Geometry check sheet. Reference: drawing and pictorial views, mm from the part's lowest x, y, z. A direction names the side the tool comes from. Coordinates: 2 decimals unless noted, no trailing zeros. Order: outer loops, then holes, each group sorted by start corner. A loop starts at its lowest first (then second) coordinate and runs counter-clockwise, first axis right, second up. Notation, with made-up numbers: (74.5, 64) -> (110.5, 64) arc R17 ccw to (110.5, 95) -> close; hole circle Ø7 at (-31.5, 80.25). An arc over 180 degrees is marked (long way). Use CSV: the item, a comma, the result in double quotes. Start each with the question number.
1) Tool access check on the marked faces 1, 2 and 3. Record the directions out of +Z, -Z, +X, -X, +Y, -Y that give a thin tool (end or side, any length) a straight path to the whole face; none if there is none.
2) Sectioned sample at A-A on z = 55.5. Give the number of separate pieces and of enclosed holes in the cut face, then the cut area to 3 significant figures.
3) Sectioned sample at C-C on x = 30. Record the boundary of the cut face in (y, z), then the cut area to 3 significant figures.
4) Scan lines: line 1 along X through (y, z) = (0.8, 19.5); line 2 along Z through (x, y) = (57.5, 2.1); line 3 along X through (y, z) = (1.25, 35.5). Record each from-to range of solid material in increasing order.
5) Sectioned sample at B-B on x = 57.5. Record the boundary of the cut face in (y, z).
6) Go/stop test with flat-tipped pins: pin 1 (4.5 mm diameter, centred on x = 55.5, z = 54, fed in from +Y); pin 2 (0.5 mm diameter, centred on y = 3.5, z = 47.5, fed in from +X); pin 3 (0.8 mm diameter, centred on y = 5, z = 26, fed in from +X). Record where each tip stops, or that it passes through.
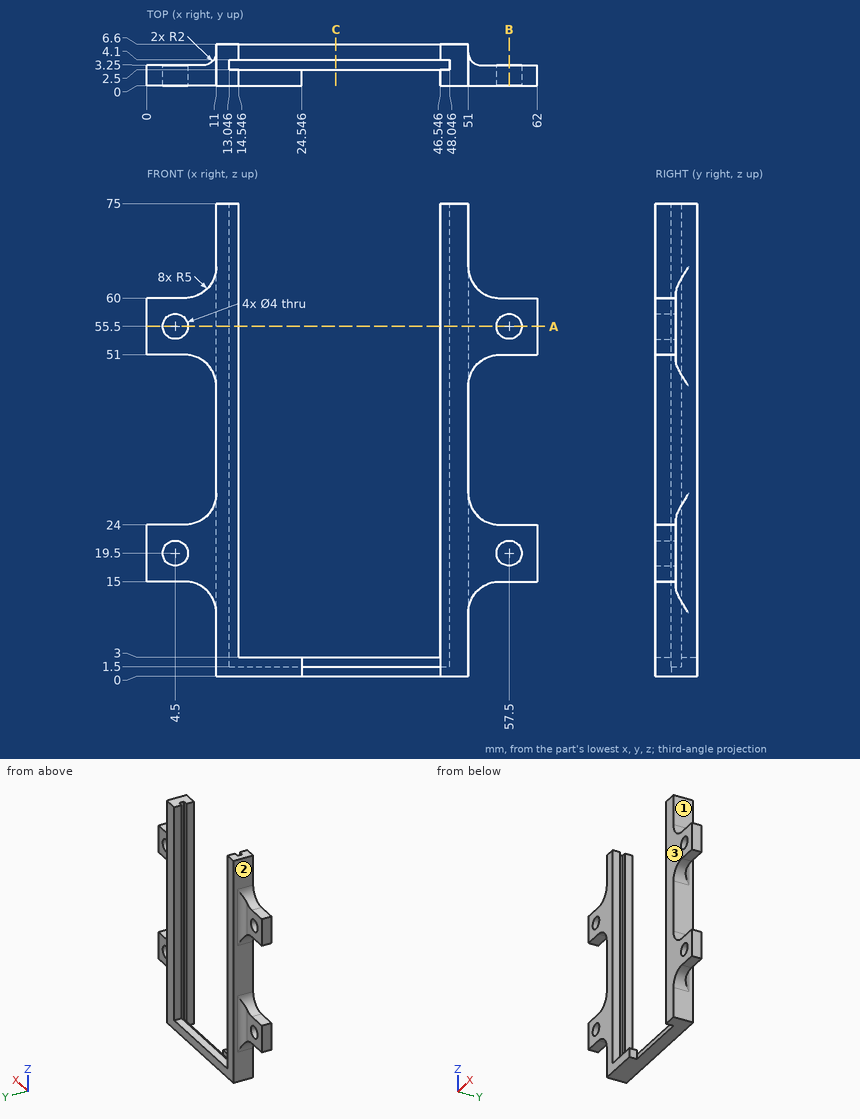
Answers follow:
1,face 1,"+X, +Y"
1,face 2,"-X, +Y"
1,face 3,"+Z, -Z, +X, -X, -Y"
2,separate pieces,"4"
2,enclosed holes,"0"
2,area,"95.2 mm²"
3,outline,"(2.5, 0) -> (6.6, 0) -> (6.6, 3) -> (4.1, 3) -> (4.1, 1.5) -> (2.5, 1.5) -> close"
3,area,"9.90 mm²"
4,line 1,"x = 0 to 2.5, 6.5 to 14.55, 46.55 to 55.5, 59.5 to 62"
4,line 2,"z = 15 to 17.5, 21.5 to 24, 51 to 53.5, 57.5 to 60"
4,line 3,"x = 11 to 14.55, 46.55 to 51"
5,outline,"(0, 15) -> (3.25, 15) -> (3.25, 17.5) -> (0, 17.5) -> close; (0, 21.5) -> (3.25, 21.5) -> (3.25, 24) -> (0, 24) -> close; (0, 51) -> (3.25, 51) -> (3.25, 53.5) -> (0, 53.5) -> close; (0, 57.5) -> (3.25, 57.5) -> (3.25, 60) -> (0, 60) -> close"
6,pin 1,"stops at y = 3.25"
6,pin 2,"stops at x = 51.32"
6,pin 3,"stops at x = 51.11"
